Here's the drawing with two shaded views (mm, measured from the low corner). I have some questions. Coordinates: 2 decimals unless noted, no trailing zeros. Loops run counter-clockwise (first coordinate to the right, second up) from the corner with the lowest first, then second, coordinate; pieces in that order, holes last. Notation, with made-up numbers: (75, 26.5) -> (104, 26.5) arc R20 ccw to (104, 37.5) -> close; hole circle Ø3 at (-23, -17.5). An arc over 180 degrees is marked (long way). Answer as a JSON object with one key per item and string values. Group by question number.
Q1. I want a section at A-A on z = 69.85. Write out the boundary of the cut face in (x, y), then the cut area to 3 significant figures.
Q2. I'm going to push a flat-ended pin straight in: pin 1 (6.5 mm diameter, centred on x = 36.5, z = 30.5, fed in from +Y). Where does the tip first touch, or does it pass through?
Q3. I need wall thicknesses on line 1 (X direction, y = 1.1, z = 69.85); line 2 (Z direction, x = 37.5, y = 5.25); line 3 (Z direction, x = 76.2, y = 3.35). Which ranges of each line are inside material? Lowest first, please.
Q4. I want a section at C-C on y = 8.75. Count the separate pieces of the cut face and the enclosed holes in it, then the cut area to 3 significant figures.
Q5. I want a section at B-B on x = 76.2. Write out the boundary of the cut face in (y, z), then the cut area to 3 significant figures.
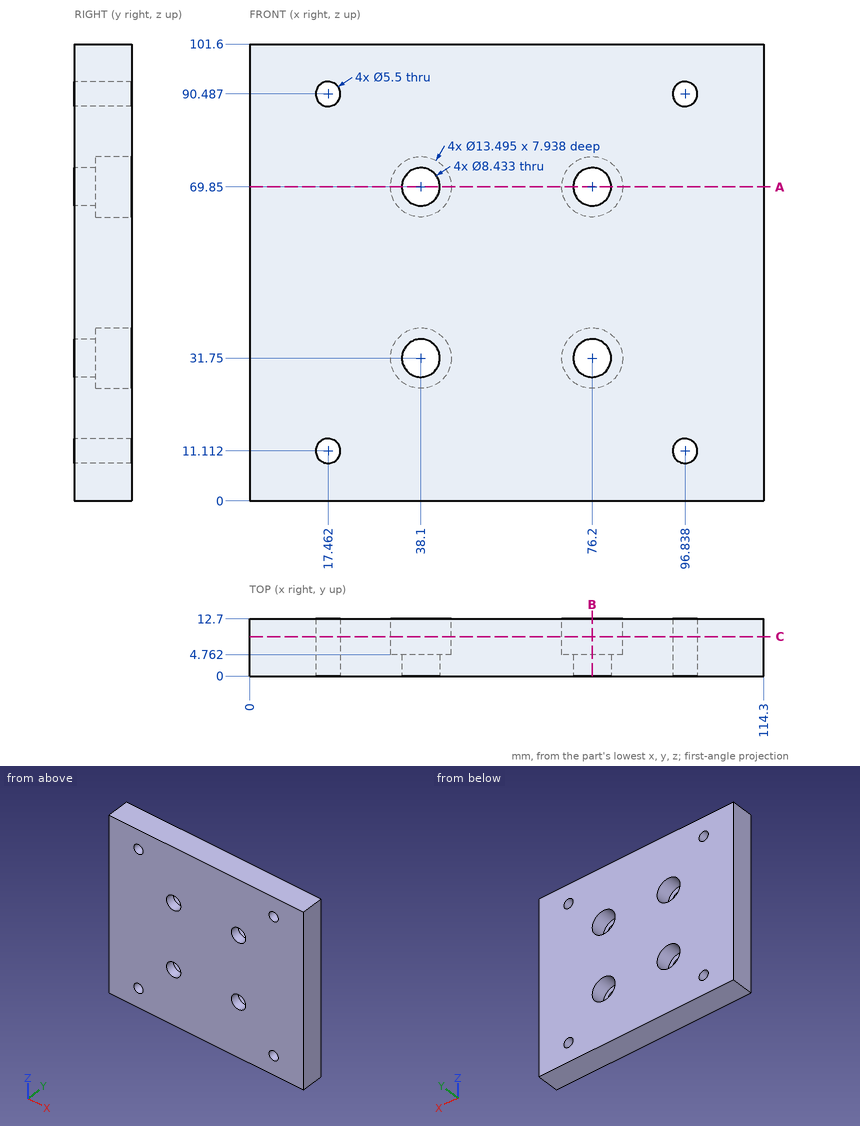
Result set:
{
 "1": {"outline": "(0, 0) -> (33.88, 0) -> (33.88, 4.76) -> (31.35, 4.76) -> (31.35, 12.7) -> (0, 12.7) -> close; (42.32, 0) -> (71.98, 0) -> (71.98, 4.76) -> (69.45, 4.76) -> (69.45, 12.7) -> (44.85, 12.7) -> (44.85, 4.76) -> (42.32, 4.76) -> close; (80.42, 0) -> (114.3, 0) -> (114.3, 12.7) -> (82.95, 12.7) -> (82.95, 4.76) -> (80.42, 4.76) -> close", "area": "1,160 mm²"},
 "2": {"pin 1": "stops at y = 4.76"},
 "3": {"line 1": "x = 0 to 33.88, 42.32 to 71.98, 80.42 to 114.3", "line 2": "z = 0 to 25.03, 38.47 to 63.13, 76.57 to 101.6", "line 3": "z = 0 to 27.53, 35.97 to 65.63, 74.07 to 101.6"},
 "4": {"separate pieces": "1", "enclosed holes": "8", "area": "10,900 mm²"},
 "5": {"outline": "(0, 0) -> (12.7, 0) -> (12.7, 25) -> (4.76, 25) -> (4.76, 27.53) -> (0, 27.53) -> close; (0, 35.97) -> (4.76, 35.97) -> (4.76, 38.5) -> (12.7, 38.5) -> (12.7, 63.1) -> (4.76, 63.1) -> (4.76, 65.63) -> (0, 65.63) -> close; (0, 74.07) -> (4.76, 74.07) -> (4.76, 76.6) -> (12.7, 76.6) -> (12.7, 101.6) -> (0, 101.6) -> close", "area": "996 mm²"}
}
